Here's how the part is built. I have some questions about the finished solid (model axes, mm). A direction names the side the tool comes from. Round coordinates to 2 decimals unless told otherwise and drop trailing zeros. Write each loop counter-clockwise with the first axis right and the second up, starting at its lowest first coordinate (ties: lowest second). Pieces come first, ordered by that corner, then holes. Notation, with made-up numbers: (48, 31) - (75, 31) arc R20 cw to (75, 47) - close; hole circle Ø4 at (-33.75, 18.25). An arc over 180 degrees is marked (long way). Write item = value, one per line. Start each with the question number.
Item 1: If we section it at A-A (z = 24): Please give me the cut outline in (x, y).
Item 2: If we section it at D-D (z = 17): Please give me the cut outline in (x, y).
Item 3: Which directions (+Z, -Z, +X, -X, +Y, -Y) give clear straight access to the entire face, cutting with the end or side of a thin tool? Please do faces 4 (the face through (0, 1, 15)), 5 (the face through (11.384, -33.549, 14.338)), 6 (the face through (5.19, 3.02, 11.06)), 7 (the face through (0, -20, 7)), 8 (the face through (20, -12, 4)).
Item 4: For P1, Ø15.5, axis at x = 0, y = 13, coming from the +Z side; P2, Ø1.5, axis at x = -7, z = 7, coming from the +Y side, each with a flat end and sliding along its axis, tell me the tip position at first contact or that it passes through.
Item 5: If we section it at C-C (x = 0): Please give me the cut outline in (y, z).
Item 6: Thinking about a two-plate mould opening in Y: for faces 1 (the face through (-10.65, -22.93, 3.55)), 2 (the face through (0, -3, 0)), 3 (the face through (0, 30, 7)), which applies, pulls with the +Y half, pulls with the -Y half, needs draft (parallel to the pull), parting line crosses it, or undercut?
Item 7: If I drill on line 1 along Y through (x, z) = (9.5, 24.5); line 2 along Z through (x, y) = (-10, -34); line 3 along Y through (x, z) = (0, 10), over which ranges is the centre line in solid material (lowest first)? Write a range as [from, to].
Item 8: If we section it at B-B (y = -20): Please give me the cut outline in (x, z), and give its area (3 significant figures).
Autodesk Inventor part; units mm, degrees
ref_plane "YZ Plane" through (0, 0, 0) normal (1, 0, 0) x (0, 1, 0)
ref_plane "XZ Plane" through (0, 0, 0) normal (0, 1, 0) x (-1, 0, 0)
ref_plane "XY Plane" through (0, 0, 0) normal (0, 0, 1) x (1, 0, 0)
sketch "Sketch1" plane through (0, 0, 0) normal (0, 0, 1) x (1, 0, 0)
  line L0 (-20, -30) -> (20, -30)
  line L1 (20, -30) -> (20, 30)
  line L2 (20, 30) -> (-20, 30)
  line L3 (-20, 30) -> (-20, -30)
  line L4 (-20, -30) -> (20, 30) construction
  line L5 (20, -30) -> (-20, 30) construction
  point P0 (0, 0)
  dimension "d0" = 40
  dimension "d1" = 60
extrude "Extrusion1" add sketch "Sketch1" along normal blind 15
sketch "Sketch2" plane through (0, 0, 15) normal (0, 0, 1) x (1, 0, 0)
  circle A0 centre (0, 13) radius 11.25
  line L0 (-20, -30) -> (20, -30)
  point P0 (0, 0)
  dimension "d4" = 22.5
  dimension "d5" = 43
extrude "Extrusion2" cut sketch "Sketch2" against normal blind 8
sketch "Sketch3" plane through (0, 13, 7) normal (0, 0, 1) x (1, 0, 0)
  circle A0 centre (0, 0) radius 6
  point P0 (0, -13)
  dimension "d8" = 12
extrude "Extrusion3" cut sketch "Sketch3" against normal through all
fillet "Fillet1" radius 16 2 edges at (20, 30, 7.5) (-20, 30, 7.5)
sketch "Sketch4" plane through (0, 0, 15) normal (0, 0, 1) x (1, 0, 0)
  line L0 (-20, 14) -> (-20, -30)
  line L1 (20, -30) -> (20, 14)
  line L2 (-20, -30) -> (20, -30)
  line L3 (20, -30) -> (20, -10)
  line L4 (20, -10) -> (-20, -10)
  line L5 (-20, -10) -> (-20, -30)
  point P0 (0, 0)
  dimension "d12" = 20
extrude "Extrusion4" cut sketch "Sketch4" against normal blind 8
sketch "Sketch5" plane through (-20, -30, 0) normal (0, -1, 0) x (1, 0, 0)
  line L0 (0, 0) -> (40, 0)
  line L1 (40, 0) -> (0, 0)
  line L2 (0, 0) -> (0, 27)
  line L3 (0, 27) -> (40, 27)
  line L4 (40, 27) -> (40, 0)
  point P0 (20, 0)
  dimension "d15" = 27
extrude "Extrusion5" add sketch "Sketch5" along normal blind 7
sketch "Sketch6" plane through (0, 0, 7) normal (0, 0, 1) x (1, 0, 0)
  circle A0 centre (-10, -20) radius 3
  circle A1 centre (10, -20) radius 3
  line L0 (20, -30) -> (-20, -30)
  line L1 (0, -42) -> (0, 42)
  point P0 (0, 0)
  dimension "d19" = 6
  dimension "d20" = 6
  dimension "d21" = 10
  dimension "d22" = 20
  dimension "d23" = 10
  dimension "d24" = 10
extrude "Extrusion6" cut sketch "Sketch6" against normal blind 7
sketch "Sketch7" plane through (-20, -37, 0) normal (0, -1, 0) x (1, 0, 0)
  circle A0 centre (30, 17) radius 3
  circle A1 centre (10, 17) radius 3
  line L0 (40, 27) -> (0, 27)
  point P0 (20, 0)
  dimension "d27" = 6
  dimension "d28" = 6
  dimension "d29" = 10
  dimension "d30" = 10
  dimension "d31" = 20
  dimension "d32" = 10
extrude "Extrusion7" cut sketch "Sketch7" against normal blind 7
sketch "Sketch8" plane through (0, 0, 15) normal (0, 0, 1) x (1, 0, 0)
  line L0 (-20, -10) -> (20, -10)
  line L1 (20, -10) -> (20, 14)
  line L2 (-20, -10) -> (20, -10)
  line L3 (20, -10) -> (20, -5)
  line L4 (20, -5) -> (-20, -5)
  line L5 (-20, -5) -> (-20, -10)
  point P0 (0, 0)
  dimension "d35" = 5
extrude "Extrusion8" add sketch "Sketch8" along normal blind 12
properties part number "Giu truc X"
Reply:
q1.outline = (-20, -37) - (20, -37) - (20, -30) - (-20, -30) - close; (-20, -10) - (20, -10) - (20, -5) - (-20, -5) - close
q2.outline = (-20, -37) - (-13, -37) - (-13, -30) - (-20, -30) - close; (-20, -10) - (20, -10) - (20, -5) - (-20, -5) - close; (-7, -37) - (7, -37) - (7, -30) - (-7, -30) - close; (13, -37) - (20, -37) - (20, -30) - (13, -30) - close
q3.face_4 = +Z, +X, -X, +Y
q3.face_5 = -Y
q3.face_6 = +Z
q3.face_7 = +Z, +X, -X
q3.face_8 = +Z, -Z, +X, +Y, -Y
q4.P1 = 7
q4.P2 = 29.84
q5.outline = (-37, 0) - (7, 0) - (7, 7) - (1.75, 7) - (1.75, 15) - (-5, 15) - (-5, 27) - (-10, 27) - (-10, 7) - (-30, 7) - (-30, 27) - (-37, 27) - close; (19, 0) - (30, 0) - (30, 15) - (24.25, 15) - (24.25, 7) - (19, 7) - close
q6.face_1 = undercut
q6.face_2 = needs draft
q6.face_3 = pulls with the +Y half
q7.line_1 = [-37, -30], [-10, -5]
q7.line_2 = [0, 14], [20, 27]
q7.line_3 = [-37, -30], [-10, 1.75], [24.25, 30]
q8.outline = (-20, 0) - (-13, 0) - (-13, 7) - (-20, 7) - close; (-7, 0) - (7, 0) - (7, 7) - (-7, 7) - close; (13, 0) - (20, 0) - (20, 7) - (13, 7) - close
q8.area = 196 mm2
